The model under review builds one solid part; all positions refer to its coordinate system, in mm. Face numbers are marked on the shaded views. Give positions to 0.01 mm unless a question says otherwise; leave off trailing zeros. Write each loop counter-clockwise with the first axis right and the second up, starting at its lowest first coordinate (ties: lowest second). Pieces come first, ordered by that corner, then holes.
from build123d import *

# Parameters (mm, degrees)
SKETCH2_R           = 0.5
BOSS_EXTRUDE1_DEPTH = 3.5


with BuildPart() as part:
    # Sketch1 → Base-Revolve (revolve)
    with BuildSketch(Plane.XY):
        with BuildLine():
            Line((-6.35, 0.1), (3.65, 0.1))
            Line((3.65, 0.1), (3.65, 0))
            Line((3.65, 0), (5.15, 0))
            ThreePointArc((5.15, 0), (5.857106781, 0.292893219), (6.15, 1))
            Line((6.15, 1), (6.15, 2.88))
            ThreePointArc((6.15, 2.88), (5.858311082, 5.020546719), (5.004514935, 7.005))
            ThreePointArc((5.004514935, 7.005), (5.858311082, 8.989453281), (6.15, 11.13))
            Line((6.15, 11.13), (6.15, 48.2))
            ThreePointArc((6.15, 48.2), (5.564213562, 49.614213562), (4.15, 50.2))
            Line((4.15, 50.2), (3.65, 50.2))
            Line((3.65, 50.2), (3.65, 50.1))
            Line((3.65, 50.1), (-6.35, 50.1))
            Line((-6.35, 50.1), (-6.35, 0.1))
        make_face()
    revolve(axis=Axis((-6.35, 50.2, 0), (0, -1, 0)))

    # Sketch2 → Boss-Extrude1 (add)
    with BuildSketch(Plane.XZ.offset(-0.1)):
        Circle(SKETCH2_R)
        with Locations((-12.7, 0)):
            Circle(SKETCH2_R)
    extrude(amount=BOSS_EXTRUDE1_DEPTH)


solid = part.part
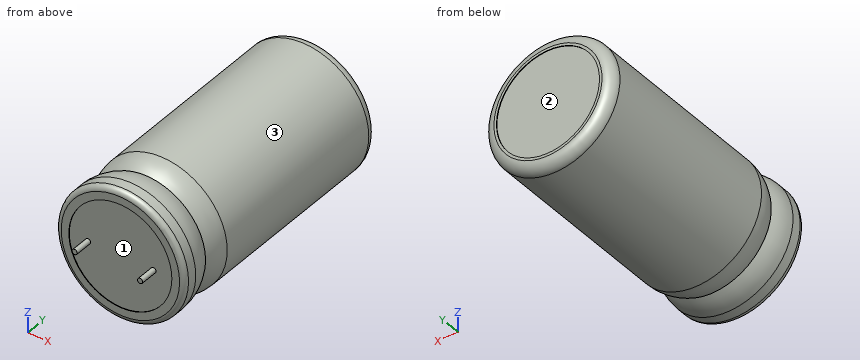
1) The part is to be moulded in two halves that separate along Z. For the marked faces 1, 2 and 3, say which applies: +Z half, -Z half, draft (parallel to the pull), parting line (faces both ways), or undercut.
2) Consider section A-A, the plane y = 37. Give the boundary of the cut face in (x, z), then the cut area to 3 significant figures.
3) Insertion check: pin 1 (1 mm diameter, centred on y = 18, z = -3, fed in from +X); pin 2 (1 mm diameter, centred on y = 27, z = -3.5, fed in from -X); pin 3 (1.5 mm diameter, centred on x = -10.5, z = 7.5, fed in from +Y); pin 4 (10 mm diameter, centred on x = -5, z = -1.5, fed in from -Y). Each pin has a flat end and moves straight along its axis. Give the tip position at first contact, or say it passes through.
4) To check wall thickness, follow probe 1 along Y at (x, z) = (-8, -0.25); probe 2 along Y at (x, z) = (-9.25, 9.75); probe 3 along Z at (x, y) = (-8.5, 1.5). State the ranges of each line that lie inside material, in increasing order.
Answer block:
1. face 1: undercut
1. face 2: undercut
1. face 3: parting line
2. outline: circle Ø25 at (-6.35, 0)
2. area: 491 mm2
3. pin 1: stops at x = 5.9
3. pin 2: stops at x = -18.48
3. pin 3: stops at y = 50.1
3. pin 4: stops at y = -3.4
4. probe 1: y = 0.1 to 50.1
4. probe 2: y = 0 to 50.2
4. probe 3: z = -12.31 to 12.31
